Geometry check sheet. Reference: the model listing, model coordinates, mm. A direction names the side the tool comes from. Give positions to 0.01 mm unless a question says otherwise; leave off trailing zeros. Write each loop counter-clockwise with the first axis right and the second up, starting at its lowest first coordinate (ties: lowest second). Pieces come first, ordered by that corner, then holes. Notation, with made-up numbers: (29, 65.5) - (71, 65.5) arc R18 cw to (71, 99.5) - close; hole circle Ø1 at (-1.5, -25). An arc over 180 degrees is marked (long way). Use a Markdown table: item, result.
```python
from build123d import *

# Parameters (mm, degrees)
F1_DEPTH = 19
F2_R     = 18.99999
F4_DEPTH = 4


# Not quite as in the source:
# - a fillet or chamfer is up to 0.001 mm smaller than in the source, because OpenCascade refuses the exact size


with BuildPart() as f1:
    # F0 (on Front) → F1 (new body, symmetric)
    with BuildSketch(Plane.XZ):
        Polygon((0, 54), (0, 0), (57, 0), (57, 11), (11, 11), (11, 54), align=None)
    extrude(amount=F1_DEPTH, both=True)

    # F2 (radius 19 in the source; OpenCascade refuses exactly that, so slightly less here)
    f2_edges = [f1.edges().sort_by_distance(p)[0] for p in [
        (5.5, -19, 54),
        (5.5, 19, 54),
        (57, -19, 5.5),
        (57, 19, 5.5),
    ]]
    fillet(f2_edges, radius=F2_R)

    # F3 (on Front) → F4 (join, symmetric)
    with BuildSketch(Plane.XZ):
        Polygon((49, 11), (11, 46), (11, 35), (11, 11), (38, 11), align=None)
    extrude(amount=F4_DEPTH, both=True)


solid = f1.part
```
1) Set-up check for faces 1 (the cylindrical face through (51.58, -13.29, 5.58)), 2 (the flat face through (11, -4.5, 32.2)), 3 (the flat face through (21, 4, 21)), 4 (the flat face through (21, -4, 21)), 5 (the cylindrical face through (51.58, 13.29, 5.58)): record each of +Z, -Z, +X, -X, +Y, -Y from which the full face is reachable in a straight line by a thin tool's end or side.
Working result:
| item | result |
|---|---|
| face 1 | +Z, -Z, +X, -Y |
| face 2 | +Z, +X, -Y |
| face 3 | +Z, +X, +Y |
| face 4 | +Z, +X, -Y |
| face 5 | +Z, -Z, +X, +Y |
2) Section check D-D on x = 20. Record the boundary of the cut face in (y, z), then the cut area to 3 significant figures.
Working result:
| item | result |
|---|---|
| outline | (-19, 0) - (19, 0) - (19, 11) - (4, 11) - (4, 37.71) - (-4, 37.71) - (-4, 11) - (-19, 11) - close |
| area | 632 mm² |
3) Material ranges on L1, parallel to Z at x = 53, y = 3; L2, parallel to Y at x = 15, z = 29.5, recorded low to high. Write a range as from..to.
Working result:
| item | result |
|---|---|
| L1 | z = 0..11 |
| L2 | y = -4..4 |
4) Section check C-C on y = -7.5. Record the boundary of the cut face in (x, z), then the cut area to 3 significant figures.
Working result:
| item | result |
|---|---|
| outline | (0, 0) - (55.46, 0) - (55.46, 11) - (11, 11) - (11, 52.46) - (0, 52.46) - close |
| area | 1,070 mm² |
5) Depth check by flat-ended pin: P1, Ø3, axis at x = 44.5, y = -1.5, coming from the +Z side; P2, Ø2, axis at y = 8.5, z = 27.5, coming from the +X side; P3, Ø4, axis at y = 5, z = 19.5, coming from the +X side. Enter the tip coordinate at first touch or a pass-through.
Working result:
| item | result |
|---|---|
| P1 | stops at z = 16.53 |
| P2 | stops at x = 11 |
| P3 | stops at x = 41.65 |
6) Section check B-B on z = 19. Record the boundary of the cut face in (x, y), then the cut area to 3 significant figures.
Working result:
| item | result |
|---|---|
| outline | (0, -19) - (11, -19) - (11, -4) - (40.31, -4) - (40.31, 4) - (11, 4) - (11, 19) - (0, 19) - close |
| area | 653 mm² |
